```python
from build123d import *

# Parameters (mm, degrees)
SKETCH_1_W          = 188
SKETCH_1_H          = 128
EXTRUDE_1_DEPTH     = 2
SKETCH_8_R          = 3.1
CUT_EXTRUDE_5_DEPTH = 1.1
SKETCH_11_W         = 164
SKETCH_11_H         = 100
CUT_EXTRUDE_8_DEPTH = 10
FILLET_2_R          = 4


with BuildPart() as part:
    # 草图1 → 凸台-拉伸1 (new body)
    with BuildSketch(Plane(origin=(0, 0, 0), x_dir=(0, 0, -1), z_dir=(1, 0, 0))):
        with Locations((-39.672025676, 38.239203457)):
            Rectangle(SKETCH_1_W, SKETCH_1_H)
    extrude(amount=EXTRUDE_1_DEPTH)

    # 草图8 → 切除-拉伸5 (cut)
    with BuildSketch(Plane(origin=(2, 0, 0), x_dir=(0, 0, -1), z_dir=(1, 0, 0))):
        with Locations((-125.672025676, 97.239203457)):
            Circle(SKETCH_8_R)
        with Locations((46.327974324, 97.239203457)):
            Circle(SKETCH_8_R)
        with Locations((-125.672025676, -20.760796543)):
            Circle(SKETCH_8_R)
        with Locations((46.327974324, -20.760796543)):
            Circle(SKETCH_8_R)
    extrude(amount=-CUT_EXTRUDE_5_DEPTH, mode=Mode.SUBTRACT)

    # 草图11 → 切除-拉伸8 (cut)
    with BuildSketch(Plane.ZY):
        with Locations((39.672025676, 38.239203457)):
            Rectangle(SKETCH_11_W, SKETCH_11_H)
    extrude(amount=-CUT_EXTRUDE_8_DEPTH, mode=Mode.SUBTRACT)

    # 圆角2
    fillet_2_edges = [part.edges().sort_by_distance(p)[0] for p in [
        (1, 88.239203457, 121.672025676),
        (1, -11.760796543, 121.672025676),
        (1, -11.760796543, -42.327974324),
        (1, 88.239203457, -42.327974324),
    ]]
    fillet(fillet_2_edges, radius=FILLET_2_R)


solid = part.part
```
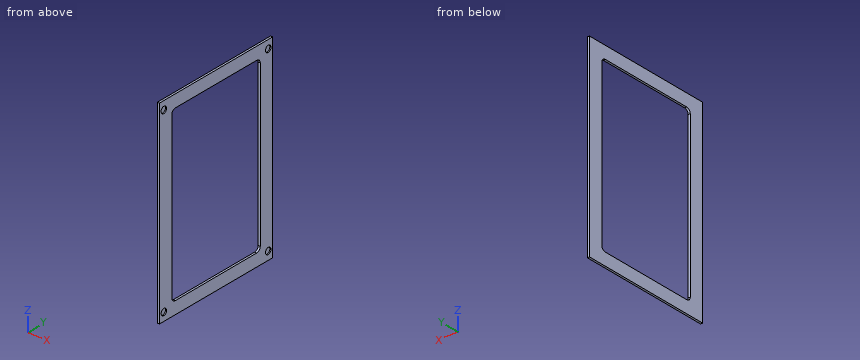
The listing builds one solid part. Answer for the finished solid, in the listing's coordinates (mm). Round coordinates to 2 decimals unless told otherwise and drop trailing zeros. Write each loop counter-clockwise with the first axis right and the second up, starting at its lowest first coordinate (ties: lowest second). Pieces come first, ordered by that corner, then holes. Notation, with made-up numbers: (89, 53.5) -> (133, 53.5) arc R21 ccw to (133, 74.5) -> close; hole circle Ø11 at (31, 30.5). An arc over 180 degrees is marked (long way). Answer as a JSON object with one key per item and string values. Group by question number.
Q1. Section A-A (y = 32) is taken. Write down the section's boundary in (x, z), plus the area to 3 significant figures.
Q2. Section B-B (z = 37.5) is taken. Write down the section's boundary in (x, y), plus the area to 3 significant figures.
Q3. Straight lines are drawn through the part: line 1 along Z through (x, y) = (1.3, 53); line 2 along Y through (x, z) = (1.4, 27.5); line 3 along Y through (x, z) = (0.6, 118). For each, find the intervals that lie inside material, in ascending order.
Q4. This flat-tipped pin is pushed along its axis until it touches: pin 1 Ø5 at (y, z) = (97.24, 125.67) entering from +X. Where does it stop, or does it pass through?
Q5. Section C-C (x = 0.45) is taken. Write down the section's boundary in (y, z).
Check values:
{
 "1": {"outline": "(0, -54.33) -> (2, -54.33) -> (2, -42.33) -> (0, -42.33) -> close; (0, 121.67) -> (2, 121.67) -> (2, 133.67) -> (0, 133.67) -> close", "area": "48.0 mm^2"},
 "2": {"outline": "(0, -25.76) -> (2, -25.76) -> (2, -11.76) -> (0, -11.76) -> close; (0, 88.24) -> (2, 88.24) -> (2, 102.24) -> (0, 102.24) -> close", "area": "56.0 mm^2"},
 "3": {"line 1": "-54.33 to -42.33, 121.67 to 133.67", "line 2": "-25.76 to -11.76, 88.24 to 102.24", "line 3": "-25.76 to -11.75, 88.23 to 102.24"},
 "4": {"pin 1": "x = 0.9"},
 "5": {"outline": "(-25.76, -54.33) -> (102.24, -54.33) -> (102.24, 133.67) -> (-25.76, 133.67) -> close; hole (-11.76, -38.33) arc R4 ccw to (-7.76, -42.33) -> (84.24, -42.33) arc R4 ccw to (88.24, -38.33) -> (88.24, 117.67) arc R4 ccw to (84.24, 121.67) -> (-7.76, 121.67) arc R4 ccw to (-11.76, 117.67) -> close"}
}
